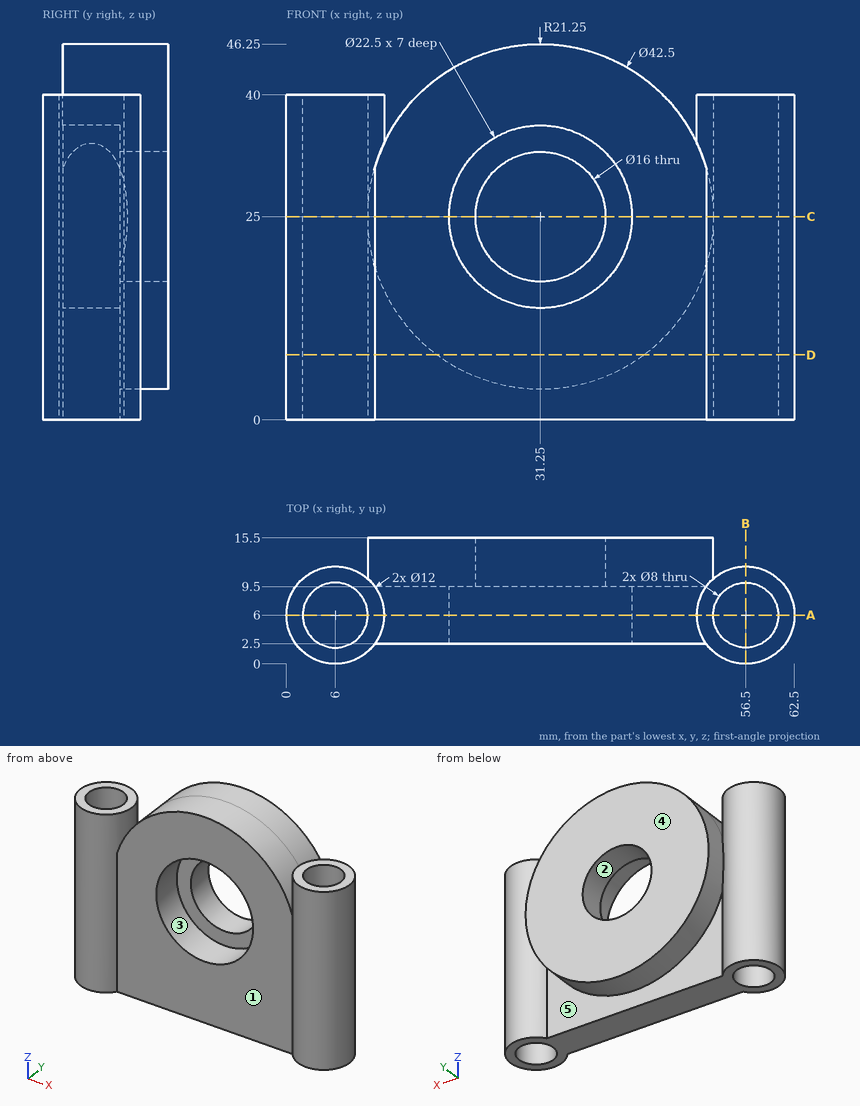
Input: dimensioned drawing with shaded views. Units: mm. Origin: part minimum x, y, z. A direction names the side the tool comes from. Round coordinates to 2 decimals unless told otherwise and drop trailing zeros. Order: outer loops, then holes, each group sorted by start corner. A loop starts at its lowest first (then second) coordinate and runs counter-clockwise, first axis right, second up. Notation, with made-up numbers: (9.25, -25) -> (43.25, -25) arc R16 cw to (43.25, 3) -> close; hole circle Ø3 at (12.25, 24.5). An arc over 180 degrees is marked (long way). One line per item, written item: value. Start each with the question number.
Q1. Draft query along X for the marked faces 4 and 5. Return one class per face: pulls with the +X half, pulls with the -X half, needs draft (parallel to the pull), parting line crosses it, or undercut.
Q2. Material intervals for probe 1 along Z at (x, y) = (31.25, 10.95); probe 2 along X at (y, z) = (9, 11); probe 3 along X at (y, z) = (6.5, 10), sorted ascending.
Q3. Pin query (flat end, axial travel): pin 1 (2 mm diameter, centred on y = 2.5, z = 23.5, fed in from +X); pin 2 (7 mm diameter, centred on x = 56.5, y = 6, fed in from +Z); pin 3 (2 mm diameter, centred on x = 14.5, z = 5, fed in from +Y); pin 4 (18 mm diameter, centred on x = 27, z = 20, fed in from -Y). Return the tip coordinate at first contact, or that it passes through.
Q4. Access query for the marked faces 1, 2 and 3. Directions: +Z, -Z, +X, -X, +Y, -Y. A direction counts if a zero-diameter tool reaches every point of the face in a straight line with its end or side. Return the directions, or none.
Q5. Section query B-B (x = 56.5). Return the cut outline in (y, z), plus the area to 3 significant figures.
Q6. Section query D-D (z = 8). Return the cut outline in (x, y).
Q7. Section query C-C (z = 25). Return the cut outline in (x, y).
Q8. Section query A-A (y = 6). Return the cut outline in (x, z), plus the area to 3 significant figures.
Findings below:
1. face 4: needs draft
1. face 5: undercut
2. probe 1: 3.75 to 17, 33 to 46.25
2. probe 2: 0.8 to 3.35, 8.65 to 53.85, 59.15 to 61.7
2. probe 3: 0.02 to 2.03, 9.97 to 52.53, 60.47 to 62.48
3. pin 1: x = 61.95
3. pin 2: through
3. pin 3: y = 9.5
3. pin 4: y = 2.5
4. face 1: +Z, -Z, -Y
4. face 2: +Y, -Y
4. face 3: -Y
5. outline: (0, 0) -> (2, 0) -> (2, 40) -> (0, 40) -> close; (10, 0) -> (12, 0) -> (12, 40) -> (10, 40) -> close
5. area: 160 mm²
6. outline: (10.87, 2.5) -> (51.63, 2.5) arc R6 ccw (long way) to (51.63, 9.5) -> (44, 9.5) -> (44, 15.5) -> (18.5, 15.5) -> (18.5, 9.5) -> (10.87, 9.5) arc R6 ccw (long way) to start; hole circle Ø8 at (6, 6); hole circle Ø8 at (56.5, 6)
7. outline: (10, 10.47) arc R6 ccw (long way) to (10.87, 2.5) -> (20, 2.5) -> (20, 9.5) -> (23.25, 9.5) -> (23.25, 15.5) -> (10, 15.5) -> close; (39.25, 9.5) -> (42.5, 9.5) -> (42.5, 2.5) -> (51.63, 2.5) arc R6 ccw (long way) to (52.5, 10.47) -> (52.5, 15.5) -> (39.25, 15.5) -> close; hole circle Ø8 at (6, 6); hole circle Ø8 at (56.5, 6)
8. outline: (0, 0) -> (2, 0) -> (2, 40) -> (0, 40) -> close; (10, 0) -> (52.5, 0) -> (52.5, 40) -> (50.5, 40) -> (50.5, 34) arc R21.25 ccw to (12, 34) -> (12, 40) -> (10, 40) -> close; (60.5, 0) -> (62.5, 0) -> (62.5, 40) -> (60.5, 40) -> close; hole circle Ø22.5 at (31.25, 25)
8. area: 1,570 mm²
